The listing builds one solid part. Answer for the finished solid, in the listing's coordinates (mm). A direction names the side the tool comes from. Give positions to 0.01 mm unless a question says otherwise; leave off trailing zeros. Order: outer loops, then holes, each group sorted by start corner. A loop starts at its lowest first (then second) coordinate and runs counter-clockwise, first axis right, second up. Notation, with made-up numbers: (56, 17.25) - (95, 17.25) arc R25 cw to (95, 45.25) - close; hole circle Ø8 at (37, 43). An arc over 180 degrees is marked (long way). Answer in a Markdown table with one row per item. Add a question column.
```python
from build123d import *

# Parameters (mm, degrees)
F1_DEPTH = 44.45
F2_DEPTH = 41.275
F4_DEPTH = 38.1


with BuildPart() as f1:
    # F0 (on Front) → F1 (new body)
    with BuildSketch(Plane.XZ):
        Polygon((0, 19.05), (0, 0), (0, -20.32), (-19.05, -20.32), (-19.05, -3.81), (-22.86, -3.81), (-22.86, -24.13), (3.81, -24.13), (3.81, 22.86), (-9.525, 22.86), (-22.86, 22.86), (-22.86, 2.54), (-19.05, 2.54), (-19.05, 19.05), align=None)
    extrude(amount=F1_DEPTH)

    # F2 (add): a face of the model
    f2_faces = [f1.faces().sort_by_distance(p)[0] for p in [
        (-9.525, -22.225, -24.13),
    ]]
    extrude(f2_faces, amount=F2_DEPTH)

    # F3 (on face) → F4 (cut)
    with BuildSketch(Plane(origin=(-22.86, 0, 0), x_dir=(0, -1, 0), z_dir=(-1, 0, 0))):
        with BuildLine():
            ThreePointArc((22.225, -33.6804), (7.9502, -47.9552), (22.225, -62.23))
            Line((22.225, -62.23), (22.225, -33.6804))
        make_face()
        with BuildLine():
            Line((22.225, -33.6804), (22.225, -62.23))
            ThreePointArc((22.225, -62.23), (32.3188078801, -58.0490078801), (36.4998, -47.9552))
            ThreePointArc((36.4998, -47.9552), (32.3188078801, -37.8613921199), (22.225, -33.6804))
        make_face()
    extrude(amount=-F4_DEPTH, mode=Mode.SUBTRACT)


solid = f1.part
```
(1) For faces 4 (the face through (-21, -22, 2.54)), 5 (the face through (-10, -44.45, -30)), 6 (the face through (-19.05, -22, -12)), determine the directions among +Z, -Z, +X, -X, +Y, -Y from which every point of the face is accessible in a straight line to the end or side of a thin tool.
(2) This flat-tipped pin is pushed along its axis until it touches: P1, Ø2, axis at y = -9.5, z = 0, coming from the -X side. Where does it stop, or does it pass through?
(3) Find section A-A, the plane x = -4.25. Write down the section's boundary in (y, z) (3 decimals).
(4) The mould has two halves that part along X. Classify faces 1 (the face through (3.81, -22, -11)), 2 (the face through (-21, -22, -3.81)), 3 (the face through (-19.05, -22, 11)): +X half, -X half, draft (parallel to the pull), parting line (faces both ways), or undercut.
(5) Find section B-B, the plane z = -7. Write down the section's boundary in (x, y), plus the area to 3 significant figures.
(6) Find section D-D, the plane y = -37.5. Write down the section's boundary in (x, z) (3 decimals).
(7) Find section C-C, the plane y = -28.5. Write down the section's boundary in (x, z) (3 decimals), plus the area to 3 significant figures.
(8) Straight lines are drawn through the part: line 1 (Z direction, x = -21.5, y = -7) (3 decimals); line 2 (Z direction, x = -13.75, y = -5) (3 decimals); line 3 (Z direction, x = -8, y = -33) (3 decimals). For each, find the intervals that lie inside material, in ascending order.
Answer key:
| question | item | result |
|---|---|---|
| 1 | face 4 | -X, +Y, -Y |
| 1 | face 5 | +Z, -Z, +X, -X, -Y |
| 1 | face 6 | +Y, -Y |
| 2 | P1 | x = 0 |
| 3 | outline | (-44.45, -65.405) - (0, -65.405) - (0, -20.32) - (-44.45, -20.32) - close; (-44.45, 19.05) - (0, 19.05) - (0, 22.86) - (-44.45, 22.86) - close; hole circle Ø28.55 at (-22.225, -47.955) |
| 4 | face 1 | +X half |
| 4 | face 2 | draft |
| 4 | face 3 | undercut |
| 5 | outline | (-22.86, -44.45) - (-19.05, -44.45) - (-19.05, 0) - (-22.86, 0) - close; (0, -44.45) - (3.81, -44.45) - (3.81, 0) - (0, 0) - close |
| 5 | area | 339 mm² |
| 6 | outline | (-22.86, -65.405) - (3.81, -65.405) - (3.81, 22.86) - (-22.86, 22.86) - (-22.86, 2.54) - (-19.05, 2.54) - (-19.05, 19.05) - (0, 19.05) - (0, -20.32) - (-19.05, -20.32) - (-19.05, -3.81) - (-22.86, -3.81) - close |
| 7 | outline | (-22.86, -65.405) - (3.81, -65.405) - (3.81, -60.777) - (-22.86, -60.777) - close; (-22.86, -35.134) - (3.81, -35.134) - (3.81, 22.86) - (-22.86, 22.86) - (-22.86, 2.54) - (-19.05, 2.54) - (-19.05, 19.05) - (0, 19.05) - (0, -20.32) - (-19.05, -20.32) - (-19.05, -3.81) - (-22.86, -3.81) - close |
| 7 | area | 896 mm² |
| 8 | line 1 | -65.405 to -3.81, 2.54 to 22.86 |
| 8 | line 2 | -65.405 to -20.32, 19.05 to 22.86 |
| 8 | line 3 | -65.405 to -57.318, -38.592 to -20.32, 19.05 to 22.86 |
